```python
from build123d import *

# Parameters (mm, degrees)
BOSS_EXTRUDE1_DEPTH            = 20
SKETCH2_R                      = 12.5
CUT_EXTRUDE1_DEPTH             = 20
CUT_EXTRUDE3_DEPTH             = 16
BOSS_EXTRUDE9_DEPTH            = 32
CUT_EXTRUDE5_OUTLINE_R         = 12.5
CUT_EXTRUDE5_DEPTH             = 20
SKETCH10_R                     = 7.5
BOSS_EXTRUDE10_DEPTH           = 6
SKETCH11_R                     = 6.5
BOSS_EXTRUDE11_DEPTH           = 5
FILLET5_R                      = 1
FILLET6_R                      = 1
CUT_EXTRUDE7_DEPTH             = 147.965990964
CUT_EXTRUDE7_DEPTH_BACK        = 147.965990964
CUT_EXTRUDE8_REACH             = 148.864
SKETCH21_R                     = 5
CUT_EXTRUDE8_DIRECTION_2_DEPTH = 147.863882558
SKETCH23_R                     = 12.5
SKETCH23_R_2                   = 5
BOSS_EXTRUDE12_DEPTH           = 22
CUT_EXTRUDE13_DEPTH            = 174.703770828
CUT_EXTRUDE13_DEPTH_BACK       = 45
SKETCH24_R                     = 3
SKETCH25_R                     = 11
SKETCH25_R_2                   = 8
BOSS_EXTRUDE13_DEPTH           = 2
BOSS_EXTRUDE14_START           = 10
SKETCH26_R                     = 11
SKETCH26_R_2                   = 3
BOSS_EXTRUDE14_DEPTH           = 10
SKETCH27_R                     = 6
SKETCH27_R_2                   = 3
BOSS_EXTRUDE15_DEPTH           = 5
CUT_EXTRUDE15_DEPTH            = 12


# Read off the part's stored shape, not the designer's step: Cut-Extrude5
with BuildPart() as part:
    # Sketch1 → Boss-Extrude1 (new body)
    with BuildSketch(Plane(origin=(0, 0, 0), x_dir=(1, 0, 0), z_dir=(0, 1, 0))):
        with BuildLine():
            Line((-90, 16), (13.288085522, 16))
            ThreePointArc((13.288085522, 16), (37.171658785, 22.533063908), (53.648380073, 4.05))
            Line((53.648380073, 4.05), (68.648380073, 4.05))
            Line((68.648380073, 4.05), (68.648380073, 0.05))
            Line((68.648380073, 0.05), (53.999946808, 0.05))
            ThreePointArc((53.999946808, 0.05), (54, 0), (53.999946808, -0.05))
            Line((53.999946808, -0.05), (68.648380073, -0.05))
            Line((68.648380073, -0.05), (68.648380073, -4.05))
            Line((68.648380073, -4.05), (53.648380073, -4.05))
            ThreePointArc((53.648380073, -4.05), (37.171658785, -22.533063908), (13.288085522, -16))
            Line((13.288085522, -16), (-90, -16))
            ThreePointArc((-90, -16), (-106, 0), (-90, 16))
        make_face()
    extrude(amount=BOSS_EXTRUDE1_DEPTH)

    # Sketch2 → Cut-Extrude1 (cut)
    with BuildSketch(Plane.XZ):
        with Locations(Location((-90, 0, 0), (0, 0, 270))):
            Circle(SKETCH2_R)
        with BuildLine():
            Line((53.999946808, -0.05), (51.99994186, -0.05))
            ThreePointArc((51.99994186, -0.05), (9, 0), (51.99994186, 0.05))
            Line((51.99994186, 0.05), (53.999946808, 0.05))
            ThreePointArc((53.999946808, 0.05), (54, 0), (53.999946808, -0.05))
        make_face()
    extrude(amount=-CUT_EXTRUDE1_DEPTH, mode=Mode.SUBTRACT)

    # Sketch3 → Cut-Extrude3 (cut)
    with BuildSketch(Plane.XZ):
        with BuildLine():
            Line((-79.416994756, -12), (10.294802649, -12))
            ThreePointArc((10.294802649, -12), (7, 0), (10.294802649, 12))
            Line((10.294802649, 12), (-79.416994756, 12))
            ThreePointArc((-79.416994756, 12), (-75.416994756, 6.583005244), (-74, 0))
            ThreePointArc((-74, 0), (-75.416994756, -6.583005244), (-79.416994756, -12))
        make_face()
    extrude(amount=-CUT_EXTRUDE3_DEPTH, mode=Mode.SUBTRACT)

    # Sketch7 → Boss-Extrude9 (add)
    with BuildSketch(Plane.XY.offset(16)):
        Polygon((-106, 78), (-35.641025641, 78), (-23, 20), (-1, 20), (-18, 98), (-106, 98), align=None)
    extrude(amount=-BOSS_EXTRUDE9_DEPTH)

    # Cut-Extrude5 outline → Cut-Extrude5 (cut)
    with BuildSketch(Plane(origin=(0, 78, 0), x_dir=(1, 0, 0), z_dir=(0, 1, 0))):
        with BuildLine():
            Line((-106, -16), (-90, -16))
            ThreePointArc((-90, -16), (-101.313708581, -11.313708417), (-106, 2.31e-07))
            Line((-106, 2.31e-07), (-106, -16))
        make_face()
        with BuildLine():
            Line((-106, 16), (-106, 2.31e-07))
            ThreePointArc((-106, 2.31e-07), (-101.313708417, 11.313708581), (-90, 16))
            Line((-90, 16), (-106, 16))
        make_face()
        with Locations((-90, 0)):
            Circle(CUT_EXTRUDE5_OUTLINE_R)
    extrude(amount=CUT_EXTRUDE5_DEPTH, mode=Mode.SUBTRACT)

    # Sketch10 → Boss-Extrude10 (add)
    with BuildSketch(Plane(origin=(0, 0, -16), x_dir=(-1, 0, 0), z_dir=(0, 0, -1))):
        with Locations(Location((24, 65, 0), (0, 0, 180))):
            Circle(SKETCH10_R)
    extrude(amount=BOSS_EXTRUDE10_DEPTH)

    # Sketch11 → Boss-Extrude11 (add)
    with BuildSketch(Plane(origin=(0, 0, -22), x_dir=(-1, 0, 0), z_dir=(0, 0, -1))):
        with Locations((24, 65)):
            Circle(SKETCH11_R)
    extrude(amount=BOSS_EXTRUDE11_DEPTH)

    # Fillet5
    fillet5_edges = [part.edges().sort_by_distance(p)[0] for p in [
        (-31.5, 65, -16),
        (-17.5, 65, -27),
        (10.294802649, 8, 12),
        (7, 0, 0),
        (10.294802649, 8, -12),
        (-34.561096053, 0, -12),
        (-79.416994756, 8, -12),
        (-74, 0, 0),
        (-79.416994756, 8, 12),
        (-34.561096053, 0, 12),
        (-34.561096053, 16, 12),
        (7, 16, 0),
        (-74, 16, 0),
    ]]
    fillet(fillet5_edges, radius=FILLET5_R)

    # Fillet6
    fillet6_edges = [part.edges().sort_by_distance(p)[0] for p in [
        (-31.5, 65, -22),
    ]]
    fillet(fillet6_edges, radius=FILLET6_R - 0.0001)  # a hair under: the kernel refuses the full size

    # Sketch20 → Cut-Extrude7 (cut, two sides: drawn at the far end of the back side and taken through both)
    with BuildSketch(Plane(origin=(0, 0, -4.05), x_dir=(-1, 0, 0), z_dir=(0, 0, -1)).offset(-CUT_EXTRUDE7_DEPTH_BACK)):
        with BuildLine():
            Line((-68.648380073, 20), (-68.648380073, 10))
            ThreePointArc((-68.648380073, 10), (-65.719447885, 17.071067812), (-58.648380073, 20))
            Line((-58.648380073, 20), (-68.648380073, 20))
        make_face()
        with BuildLine():
            Line((-68.648380073, 0), (-58.648380073, 0))
            ThreePointArc((-58.648380073, 0), (-65.719447885, 2.928932188), (-68.648380073, 10))
            Line((-68.648380073, 10), (-68.648380073, 0))
        make_face()
        with BuildLine():
            ThreePointArc((-65.648380073, 10), (-59.648380073, 4), (-53.648380073, 10))
            Line((-53.648380073, 10), (-65.648380073, 10))
        make_face()
        with BuildLine():
            Line((-65.648380073, 10), (-53.648380073, 10))
            ThreePointArc((-53.648380073, 10), (-59.648380073, 16), (-65.648380073, 10))
        make_face()
    extrude(amount=CUT_EXTRUDE7_DEPTH + CUT_EXTRUDE7_DEPTH_BACK, mode=Mode.SUBTRACT)

    # Sketch21 → Cut-Extrude8 (cut, up to next)
    with BuildSketch(Plane(origin=(0, 98, 0), x_dir=(1, 0, 0), z_dir=(0, 1, 0)), mode=Mode.PRIVATE) as cut_extrude8_sk1:
        with Locations((-43, 0)):
            Circle(SKETCH21_R)
    cut_extrude8_tool1 = extrude(cut_extrude8_sk1.sketch, amount=-CUT_EXTRUDE8_REACH, mode=Mode.PRIVATE) & part.part
    add(cut_extrude8_tool1.solids().sort_by_distance((-43, 98, 0))[0], mode=Mode.SUBTRACT)

    # Sketch21 → Cut-Extrude8 direction 2 (cut)
    with BuildSketch(Plane(origin=(0, 98, 0), x_dir=(1, 0, 0), z_dir=(0, 1, 0))):
        with Locations((-43, 0)):
            Circle(SKETCH21_R)
    extrude(amount=CUT_EXTRUDE8_DIRECTION_2_DEPTH, mode=Mode.SUBTRACT)



with BuildPart() as body_2:
    # Sketch23 → Boss-Extrude12 (new body)
    with BuildSketch(Plane(origin=(0, 98, 0), x_dir=(1, 0, 0), z_dir=(0, 1, 0))):
        with BuildLine():
            Line((-118, -1.5), (-118, -16))
            Line((-118, -16), (-90, -16))
            Line((-90, -16), (-18, -16))
            Line((-18, -16), (-18, 16))
            Line((-18, 16), (-90, 16))
            Line((-90, 16), (-118, 16))
            Line((-118, 16), (-118, 1.5))
            Line((-118, 1.5), (-105.929532322, 1.5))
            ThreePointArc((-105.929532322, 1.5), (-106, 0), (-105.929532322, -1.5))
            Line((-105.929532322, -1.5), (-118, -1.5))
        make_face()
        with Locations(Location((-90, 0, 0), (0, 0, 90))):
            Circle(SKETCH23_R, mode=Mode.SUBTRACT)
        with Locations((-43, 0)):
            Circle(SKETCH23_R_2, mode=Mode.SUBTRACT)
    extrude(amount=BOSS_EXTRUDE12_DEPTH)

    # Sketch24 → Cut-Extrude13 (cut, two sides: drawn at the far end of the back side and taken through both)
    with BuildSketch(Plane.XY.offset(16).offset(-CUT_EXTRUDE13_DEPTH_BACK)):
        with BuildLine():
            ThreePointArc((-118, 109), (-114.778174593, 116.778174593), (-107, 120))
            Line((-107, 120), (-118, 120))
            Line((-118, 120), (-118, 109))
        make_face()
        with BuildLine():
            Line((-118, 98), (-107, 98))
            ThreePointArc((-107, 98), (-114.778174593, 101.221825407), (-118, 109))
            Line((-118, 109), (-118, 98))
        make_face()
        Polygon((-22.794871795, 120), (-18, 98), (-18, 120), align=None)
        with Locations(Location((-107, 109, 0), (0, 0, 180))):
            Circle(SKETCH24_R)
    extrude(amount=CUT_EXTRUDE13_DEPTH + CUT_EXTRUDE13_DEPTH_BACK, mode=Mode.SUBTRACT)


with BuildPart() as part_1:
    add(part.part)

    add(body_2.part)  # Boss-Extrude13 merges body 2
    # Sketch25 → Boss-Extrude13 (add)
    with BuildSketch(Plane.XY.offset(16)):
        with Locations(Location((-107, 109, 0), (0, 0, 270))):
            Circle(SKETCH25_R)
        with Locations((-107, 109)):
            Circle(SKETCH25_R_2, mode=Mode.SUBTRACT)
    extrude(amount=BOSS_EXTRUDE13_DEPTH)

    # Sketch26 → Boss-Extrude14 (add)
    with BuildSketch(Plane(origin=(0, 0, -16), x_dir=(-1, 0, 0), z_dir=(0, 0, -1)).offset(BOSS_EXTRUDE14_START)):
        with Locations(Location((107, 109, 0), (0, 0, 270))):
            Circle(SKETCH26_R)
        with Locations((107, 109)):
            Circle(SKETCH26_R_2, mode=Mode.SUBTRACT)
    extrude(amount=-BOSS_EXTRUDE14_DEPTH)

    # Sketch27 → Boss-Extrude15 (add)
    with BuildSketch(Plane(origin=(0, 0, -26), x_dir=(-1, 0, 0), z_dir=(0, 0, -1))):
        with Locations((107, 109)):
            Circle(SKETCH27_R)
        with Locations((107, 109)):
            Circle(SKETCH27_R_2, mode=Mode.SUBTRACT)
    extrude(amount=BOSS_EXTRUDE15_DEPTH)

    # Sketch29 → Cut-Extrude15 (cut)
    with BuildSketch(Plane.XY.offset(16)):
        Polygon((-104, 114.196152423), (-110, 114.196152423), (-113, 109), (-110, 103.803847577), (-104, 103.803847577), (-101, 109), align=None)
    extrude(amount=-CUT_EXTRUDE15_DEPTH, mode=Mode.SUBTRACT)

    # SurfaceCut1
    split(bisect_by=Plane(origin=(0, 98, 0), x_dir=(1, 0, 0), z_dir=(0, 1, 0)), keep=Keep.TOP)


solid = part_1.part
```
Verification items for the finished model (mm, model axes). A direction names the side the tool comes from. Coordinates: 2 decimals unless noted, no trailing zeros. Write each loop counter-clockwise with the first axis right and the second up, starting at its lowest first coordinate (ties: lowest second). Pieces come first, ordered by that corner, then holes. Notation, with made-up numbers: M 87,79 L 136,79 A9 ccw 136,88 Z; hole C 70,-34.75 d6. An arc over 180 degrees is marked long. Answer as a JSON object with one key per item and string values. Group by question number.
(1) Release check for a two-part mould opening along Z. For faces 1 (the face through (-108, 112, -31)), 2 (the face through (-56, 120, 0)), 3 (the face through (-112, 109, -1.5)), 4 (the face through (-106, 116, 0)) record: +Z half, -Z half, draft (parallel to the pull), parting line (faces both ways), or undercut.
(2) Cross-section at C-C, the plane z = 0. Record the cut outline in (x, y), and give its area (3 significant figures).
(3) Cross-section at B-B, the plane z = -6.5. Record the cut outline in (x, y).
(4) Cross-section at D-D, the plane x = -94.5. Record the cut outline in (y, z), and give its area (3 significant figures).
(5) Tool access check on faces 5 (the face through (-102.58, 113.06, -28.46)), 6 (the face through (-107, 103.804, 10)), 7 (the face through (-20.43, 109.15, -0.22)). Record the directions out of +Z, -Z, +X, -X, +Y, -Y that give a thin tool (end or side, any length) a straight path to the whole face; none if there is none.
(6) Gauge pin test, flat ends, axial feed: pin 1 (3 mm diameter, centred on x = -49.5, y = 110.5, fed in from +Z); pin 2 (5.5 mm diameter, centred on x = -107, y = 109, fed in from +Z); pin 3 (4 mm diameter, centred on x = -80.5, y = 113.5, fed in from -Z); pin 4 (1 mm diameter, centred on y = 103.5, z = 4.5, fed in from -X). Record the tip position at first contact, or that the pin passes through.
(7) Cross-section at A-A, the plane x = -43. Record the cut outline in (y, z), and give its area (3 significant figures).
(8) Material ranges on line 1 (Z direction, x = -43, y = 103.75); line 2 (Y direction, x = -107, z = -18); line 3 (Y direction, x = -107, z = -29.9), recorded low to high.
Reply:
{
 "1": {"face 1": "-Z half", "face 2": "draft", "face 3": "undercut", "face 4": "undercut"},
 "2": {"outline": "M -106,98 L -102.5,98 L -102.5,120 L -106,120 L -106,111.83 A3 cw -106,106.17 Z; M -77.5,98 L -48,98 L -48,120 L -77.5,120 Z; M -38,98 L -18,98 L -22.79,120 L -38,120 Z", "area": "1,110 mm²"},
 "3": {"outline": "M -107,98 L -100.68,98 L -100.68,120 L -107,120 A11 ccw Z; M -79.32,98 L -18,98 L -22.79,120 L -79.32,120 Z; hole C -107,109 d6"},
 "4": {"outline": "M 98,-16 L 120,-16 L 120,-11.66 L 98,-11.66 Z; M 98,11.66 L 120,11.66 L 120,16 L 98,16 Z", "area": "191 mm²"},
 "5": {"face 5": "-Z", "face 6": "+Z", "face 7": "+Z, -Z, +X, +Y"},
 "6": {"pin 1": "z = 16", "pin 2": "through", "pin 3": "z = -16", "pin 4": "x = -116.8"},
 "7": {"outline": "M 98,-16 L 120,-16 L 120,-5 L 98,-5 Z; M 98,5 L 120,5 L 120,16 L 98,16 Z", "area": "484 mm²"},
 "8": {"line 1": "-16 to -5, 5 to 16", "line 2": "98 to 106, 112 to 120", "line 3": "103 to 106, 112 to 115"}
}
